```python
from build123d import *

# Parameters (mm, degrees)
F0_W     = 53.34
F0_H     = 69.85
F1_DEPTH = 6.35


with BuildPart() as f1:
    # F0 (on Front) → F1 (new body)
    with BuildSketch(Plane.XZ):
        with Locations((18.915267, 5.530364)):
            Rectangle(F0_W, F0_H)
        Polygon((23.995267, 25.834043), (23.995267, 5.530364), (23.995267, -12.249636), (23.995267, -22.409636), (13.835267, -22.409636), (13.835267, -12.249636), (13.835267, 5.530364), (13.835267, 23.310364), (13.835267, 25.834043), (13.835267, 35.994043), (23.995267, 35.994043), align=None, mode=Mode.SUBTRACT)
    extrude(amount=F1_DEPTH)


solid = f1.part
```
Verification items for the finished model (mm, model axes). A direction names the side the tool comes from. Give positions to 0.01 mm unless a question says otherwise; leave off trailing zeros. Loops run counter-clockwise (first coordinate to the right, second up) from the corner with the lowest first, then second, coordinate; pieces in that order, holes last. Notation, with made-up numbers: M 78,73.25 L 102,73.25 A23 cw 102,96.25 Z; hole C 41,70 d4. An arc over 180 degrees is marked long. One line per question, with ' | ' between items.
Item 1: Tool access check on faces 4 (the face through (45.585, -3, 5)), 5 (the face through (23.995, -3, 7)). Record the directions out of +Z, -Z, +X, -X, +Y, -Y that give a thin tool (end or side, any length) a straight path to the whole face; none if there is none.
Completed:
face 4: +Z, -Z, +X, +Y, -Y | face 5: +Y, -Y
Item 2: Section check C-C, the plane y = -3.25. Record the cut outline in (x, z).
Completed:
outline: M -7.75,-29.39 L 45.59,-29.39 L 45.59,40.46 L -7.75,40.46 Z; hole M 13.84,-22.41 L 24,-22.41 L 24,35.99 L 13.84,35.99 Z
Item 3: Draft check along Z on faces 1 (the face through (-7.755, -3, 5)), 2 (the face through (13.835, -3, 6)), 3 (the face through (19, -3, 40.455)). Enter one of: +Z half, -Z half, draft (parallel to the pull), parting line (faces both ways), or undercut.
Completed:
face 1: draft | face 2: undercut | face 3: +Z half
Item 4: Section check B-B, the plane z = -19.5. Record the cut outline in (x, y), plus the area to 3 significant figures.
Completed:
outline: M -7.75,-6.35 L 13.84,-6.35 L 13.84,0 L -7.75,0 Z; M 24,-6.35 L 45.59,-6.35 L 45.59,0 L 24,0 Z | area: 274 mm^2
Item 5: Section check A-A, the plane x = 16. Record the cut outline in (y, z), plus the area to 3 significant figures.
Completed:
outline: M -6.35,-29.39 L 0,-29.39 L 0,-22.41 L -6.35,-22.41 Z; M -6.35,35.99 L 0,35.99 L 0,40.46 L -6.35,40.46 Z | area: 72.7 mm^2
Item 6: Thickness scan on line 1 (X direction, y = -2.25, z = -1.5); line 2 (Z direction, x = 21.5, y = -4.75). Record the ranges inside material, lowest first. Write a range as [from, to].
Completed:
line 1: x = [-7.75, 13.84], [24, 45.59] | line 2: z = [-29.39, -22.41], [35.99, 40.46]
